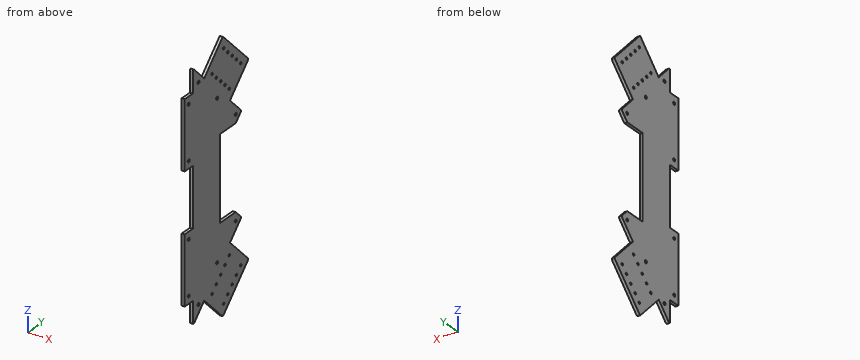
```python
from build123d import *

# Parameters (mm, degrees)
SKETCH_1_R      = 2.5
SKETCH_1_R_2    = 2
EXTRUDE_1_DEPTH = 5
FILLET_1_R      = 2


with BuildPart() as part:
    # 草图1 → 凸台-拉伸1 (new body)
    with BuildSketch(Plane(origin=(0, 0, 0), x_dir=(0, 0, -1), z_dir=(1, 0, 0))):
        Polygon((165, 0), (205, 0), (176.715728753, 28.284271247), (222.67766953, 74.246212025), (159.038059223, 137.885822331), (113.076118446, 91.923881554), (84.791847198, 120.208152802), (70.649711575, 106.066017178), (70.649711575, 67.772939569), (-70.649711575, 67.772939569), (-70.649711575, 106.066017178), (-84.791847198, 120.208152802), (-113.076118446, 91.923881554), (-159.038059223, 137.885822331), (-222.67766953, 74.246212025), (-176.715728753, 28.284271247), (-205, 0), (-165, 0), (-165, -20), (-50, -20), (-50, 0), (50, 0), (50, -20), (165, -20), align=None)
        with Locations((-176.715728753, 14.142135624)):
            Circle(SKETCH_1_R, mode=Mode.SUBTRACT)
        with Locations((-174.9479618, 47.72970773)):
            Circle(SKETCH_1_R_2, mode=Mode.SUBTRACT)
        with Locations((-164.341360082, 58.336309448)):
            Circle(SKETCH_1_R_2, mode=Mode.SUBTRACT)
        with Locations((176.715728753, 14.142135624)):
            Circle(SKETCH_1_R, mode=Mode.SUBTRACT)
        with Locations((164.341360082, 58.336309448)):
            Circle(SKETCH_1_R_2, mode=Mode.SUBTRACT)
        with Locations((174.9479618, 47.72970773)):
            Circle(SKETCH_1_R_2, mode=Mode.SUBTRACT)
        with Locations((-203.232233047, 76.013978978)):
            Circle(SKETCH_1_R_2, mode=Mode.SUBTRACT)
        with Locations((-130.753787975, 60.104076401)):
            Circle(SKETCH_1_R, mode=Mode.SUBTRACT)
        with Locations((-153.734758364, 68.942911166)):
            Circle(SKETCH_1_R_2, mode=Mode.SUBTRACT)
        with Locations((-192.625631329, 86.620580695)):
            Circle(SKETCH_1_R_2, mode=Mode.SUBTRACT)
        with Locations((-182.019029611, 97.227182413)):
            Circle(SKETCH_1_R_2, mode=Mode.SUBTRACT)
        with Locations((-143.128156646, 79.549512883)):
            Circle(SKETCH_1_R_2, mode=Mode.SUBTRACT)
        with Locations((-132.521554928, 90.156114601)):
            Circle(SKETCH_1_R_2, mode=Mode.SUBTRACT)
        with Locations((-171.412427894, 107.833784131)):
            Circle(SKETCH_1_R_2, mode=Mode.SUBTRACT)
        with Locations((-160.805826176, 118.440385849)):
            Circle(SKETCH_1_R_2, mode=Mode.SUBTRACT)
        with Locations((-84.791847198, 106.066017178)):
            Circle(SKETCH_1_R, mode=Mode.SUBTRACT)
        with Locations((130.753787975, 60.104076401)):
            Circle(SKETCH_1_R, mode=Mode.SUBTRACT)
        with Locations((153.734758364, 68.942911166)):
            Circle(SKETCH_1_R_2, mode=Mode.SUBTRACT)
        with Locations((203.232233047, 76.013978978)):
            Circle(SKETCH_1_R_2, mode=Mode.SUBTRACT)
        with Locations((143.128156646, 79.549512883)):
            Circle(SKETCH_1_R_2, mode=Mode.SUBTRACT)
        with Locations((132.521554928, 90.156114601)):
            Circle(SKETCH_1_R_2, mode=Mode.SUBTRACT)
        with Locations((192.625631329, 86.620580695)):
            Circle(SKETCH_1_R_2, mode=Mode.SUBTRACT)
        with Locations((182.019029611, 97.227182413)):
            Circle(SKETCH_1_R_2, mode=Mode.SUBTRACT)
        with Locations((84.791847198, 106.066017178)):
            Circle(SKETCH_1_R, mode=Mode.SUBTRACT)
        with Locations((171.412427894, 107.833784131)):
            Circle(SKETCH_1_R_2, mode=Mode.SUBTRACT)
        with Locations((160.805826176, 118.440385849)):
            Circle(SKETCH_1_R_2, mode=Mode.SUBTRACT)
        with Locations((152.5, -10)):
            Circle(SKETCH_1_R, mode=Mode.SUBTRACT)
        with Locations((62.5, -10)):
            Circle(SKETCH_1_R, mode=Mode.SUBTRACT)
        with Locations((-62.5, -10)):
            Circle(SKETCH_1_R, mode=Mode.SUBTRACT)
        with Locations((-152.5, -10)):
            Circle(SKETCH_1_R, mode=Mode.SUBTRACT)
    extrude(amount=EXTRUDE_1_DEPTH)

    # 圆角1
    fillet_1_edges = [part.edges().sort_by_distance(p)[0] for p in [
        (2.5, 137.885822331, -159.038059223),
        (2.5, 74.246212025, -222.67766953),
        (2.5, 0, -205),
        (2.5, 0, 205),
        (2.5, 74.246212025, 222.67766953),
        (2.5, 137.885822331, 159.038059223),
        (2.5, 120.208152802, 84.791847198),
        (2.5, 120.208152802, -84.791847198),
    ]]
    fillet(fillet_1_edges, radius=FILLET_1_R)


solid = part.part
```
Could you check a few things on this model? Use its own coordinates, in mm. Coordinates: 2 decimals unless noted, no trailing zeros. Order: outer loops, then holes, each group sorted by start corner. A loop starts at its lowest first (then second) coordinate and runs counter-clockwise, first axis right, second up. Notation, with made-up numbers: M 18.25,-38 L 32.25,-38 A30 cw 32.25,-7 Z; hole C -21,56.5 d3. An arc over 180 degrees is marked long. Use a Markdown table: item, result. Add a question column.
Q1. I'm going to push flat-ended pins straight in: pin 1 (3 mm diameter, centred on x = 4, y = 16, fed in from +Z); pin 2 (1.5 mm diameter, centred on x = 3, y = -14, fed in from -Z); pin 3 (2.5 mm diameter, centred on x = 2.5, y = 81, fed in from +Z); pin 4 (3.5 mm diameter, centred on y = 107.83, z = -171.41, fed in from -X). Where does each tip first touch, or does it pass through?
Q2. If I drill on L1, parallel to Z at x = 0.95, y = 112.5; L2, parallel to Y at x = 1.3, z = -153.5; L3, parallel to Z at x = 2.45, y = 85, over which ranges is the centre line in solid material (lowest first)?
Q3. I want a section at B-B on x = 2.55. Give the number of separate pieces and of enclosed holes in the cut face, then the cut area to 3 significant figures.
Q4. I want a section at A-A on z = -107. List the corners of the cut face in (x, y) for me, then the cut area to 3 significant figures.
Checked values:
| question | item | result |
|---|---|---|
| 1 | pin 1 | z = 190.5 |
| 1 | pin 2 | z = -165 |
| 1 | pin 3 | z = 217.17 |
| 1 | pin 4 | through |
| 2 | L1 | -184.42 to -133.65, -92.5 to -77.08, 77.08 to 92.5, 133.65 to 184.42 |
| 2 | L2 | -20 to -12.29, -7.71 to 66.96, 70.93 to 132.35 |
| 2 | L3 | -211.92 to -193.8, -191.45 to -70.65, 70.65 to 191.45, 193.8 to 211.92 |
| 3 | separate pieces | 1 |
| 3 | enclosed holes | 30 |
| 3 | area | 43,100 mm² |
| 4 | outline | M 0,-20 L 5,-20 L 5,98 L 0,98 Z |
| 4 | area | 590 mm² |
